```python
from build123d import *

# Parameters (mm, degrees)
EXTRUDE_1_DEPTH     = 58.3
CUT_EXTRUDE_1_DEPTH = 6.8
CUT_EXTRUDE_2_DEPTH = 54.3
SKETCH_5_R          = 2
CUT_EXTRUDE_4_DEPTH = 55
CHAMFER_2_SIZE      = 1
SKETCH_7_R          = 3.25
CUT_EXTRUDE_5_DEPTH = 1
SKETCH_8_R          = 1.25
CUT_EXTRUDE_6_DEPTH = 10
SKETCH_9_R          = 1
CUT_EXTRUDE_7_DEPTH = 10
SKETCH_11_W         = 6
SKETCH_11_H         = 1.5
CUT_EXTRUDE_8_DEPTH = 10


with BuildPart() as part:
    # Эскиз1 → Бобышка-Вытянуть1 (new body)
    with BuildSketch(Plane.XY):
        with BuildLine():
            Line((-3.4, 9.15), (3.4, 9.15))
            ThreePointArc((3.4, 9.15), (6.935533906, 7.685533906), (8.4, 4.15))
            Line((8.4, 4.15), (8.4, -4.15))
            Line((8.4, -4.15), (-8.4, -4.15))
            Line((-8.4, -4.15), (-8.4, 4.15))
            ThreePointArc((-8.4, 4.15), (-6.935533906, 7.685533906), (-3.4, 9.15))
        make_face()
    extrude(amount=EXTRUDE_1_DEPTH)

    # Эскиз2 → Вырез-Вытянуть1 (cut)
    with BuildSketch(Plane(origin=(0, 9.15, 0), x_dir=(1, 0, 0), z_dir=(0, 1, 0))):
        with BuildLine():
            Line((8.4, -19.65), (8.4, -2))
            Line((8.4, -2), (-8.4, -2))
            Line((-8.4, -2), (-8.4, -19.65))
            Line((-8.4, -19.65), (-6, -19.65))
            ThreePointArc((-6, -19.65), (-4.585786438, -20.235786438), (-4, -21.65))
            Line((-4, -21.65), (-4, -36.65))
            ThreePointArc((-4, -36.65), (-4.585786438, -38.064213562), (-6, -38.65))
            Line((-6, -38.65), (-8.4, -38.65))
            Line((-8.4, -38.65), (-8.4, -56.3))
            Line((-8.4, -56.3), (8.4, -56.3))
            Line((8.4, -56.3), (8.4, -38.65))
            Line((8.4, -38.65), (6, -38.65))
            ThreePointArc((6, -38.65), (4.585786438, -38.064213562), (4, -36.65))
            Line((4, -36.65), (4, -21.65))
            ThreePointArc((4, -21.65), (4.585786438, -20.235786438), (6, -19.65))
            Line((6, -19.65), (8.4, -19.65))
        make_face()
    extrude(amount=-CUT_EXTRUDE_1_DEPTH, mode=Mode.SUBTRACT)

    # Эскиз3 → Вырез-Вытянуть2 (cut)
    with BuildSketch(Plane(origin=(0, 0, 56.3), x_dir=(-1, 0, 0), z_dir=(0, 0, -1))):
        with BuildLine():
            Line((-7.4, 4.15), (-7.4, -3.15))
            Line((-7.4, -3.15), (7.4, -3.15))
            Line((7.4, -3.15), (7.4, 4.15))
            ThreePointArc((7.4, 4.15), (6.228427125, 6.978427125), (3.4, 8.15))
            Line((3.4, 8.15), (-3.4, 8.15))
            ThreePointArc((-3.4, 8.15), (-6.228427125, 6.978427125), (-7.4, 4.15))
        make_face()
    extrude(amount=CUT_EXTRUDE_2_DEPTH, mode=Mode.SUBTRACT)

    # Эскиз5 → Вырез-Вытянуть4 (cut)
    with BuildSketch(Plane(origin=(0, -3.15, 0), x_dir=(1, 0, 0), z_dir=(0, 1, 0))):
        with Locations(Location((0, -29.15, 0), (0, 0, 270))):
            Circle(SKETCH_5_R)
    extrude(amount=-CUT_EXTRUDE_4_DEPTH, mode=Mode.SUBTRACT)

    # Фаска2
    chamfer_2_edges = [part.edges().sort_by_distance(p)[0] for p in [
        (0, -3.15, 27.15),
    ]]
    chamfer(chamfer_2_edges, length=CHAMFER_2_SIZE - 0.0001)  # a hair under: the kernel refuses the full size

    # Эскиз7 → Вырез-Вытянуть5 (cut)
    with BuildSketch(Plane(origin=(0, 0, 0), x_dir=(-1, 0, 0), z_dir=(0, 0, -1))):
        with Locations((0, 3.85)):
            Circle(SKETCH_7_R)
    cut_extrude_5 = extrude(amount=-CUT_EXTRUDE_5_DEPTH, mode=Mode.SUBTRACT)

    # Эскиз8 → Вырез-Вытянуть6 (cut)
    with BuildSketch(Plane(origin=(0, 0, 0), x_dir=(-1, 0, 0), z_dir=(0, 0, -1))):
        with Locations((0, 3.85)):
            Circle(SKETCH_8_R)
    cut_extrude_6 = extrude(amount=-CUT_EXTRUDE_6_DEPTH, mode=Mode.SUBTRACT)

    # Эскиз9 → Вырез-Вытянуть7 (cut)
    with BuildSketch(Plane(origin=(0, 0, 0), x_dir=(-1, 0, 0), z_dir=(0, 0, -1))):
        with Locations((-5.4, -1.65)):
            Circle(SKETCH_9_R)
    cut_extrude_7 = extrude(amount=-CUT_EXTRUDE_7_DEPTH, mode=Mode.SUBTRACT)

    # Эскиз11 → Вырез-Вытянуть8 (cut)
    with BuildSketch(Plane(origin=(0, -3.15, 0), x_dir=(1, 0, 0), z_dir=(0, 1, 0))):
        with Locations((0, -2.75)):
            Rectangle(SKETCH_11_W, SKETCH_11_H)
    cut_extrude_8 = extrude(amount=-CUT_EXTRUDE_8_DEPTH, mode=Mode.SUBTRACT)

    # Зеркальное отражение1: Вырез-Вытянуть5, Вырез-Вытянуть6, Вырез-Вытянуть7, Вырез-Вытянуть8 across plane
    add(cut_extrude_5.mirror(Plane(origin=(0, 0, 29.15), x_dir=(1, 0, 0), z_dir=(0, 0, -1))), mode=Mode.SUBTRACT)
    add(cut_extrude_6.mirror(Plane(origin=(0, 0, 29.15), x_dir=(1, 0, 0), z_dir=(0, 0, -1))), mode=Mode.SUBTRACT)
    add(cut_extrude_7.mirror(Plane(origin=(0, 0, 29.15), x_dir=(1, 0, 0), z_dir=(0, 0, -1))), mode=Mode.SUBTRACT)
    add(cut_extrude_8.mirror(Plane(origin=(0, 0, 29.15), x_dir=(1, 0, 0), z_dir=(0, 0, -1))), mode=Mode.SUBTRACT)


solid = part.part
```
Work out the finished part from the listing and answer in its coordinate system (mm). A direction names the side the tool comes from. Round coordinates to 2 decimals unless told otherwise and drop trailing zeros. Loops run counter-clockwise (first coordinate to the right, second up) from the corner with the lowest first, then second, coordinate; pieces in that order, holes last. Notation, with made-up numbers: (75, -3.75) -> (100, -3.75) arc R25 cw to (100, 31.25) -> close; hole circle Ø7 at (15.5, -10.5). An arc over 180 degrees is marked (long way). Write each question's results on one line, items separated by ' | '. Start each with the question number.
1. Find the intervals of material crossed by probe 1 along Z at (x, y) = (-7.5, 6.5); probe 2 along X at (y, z) = (3.85, 56.7); probe 3 along Y at (x, z) = (0, 0.7), in increasing order. Write a range as from..to.
2. For a pull along X with two mould halves and no side action, classify faces 6 (the face through (-8, 2.35, 11)), 7 (the face through (6.9, 7.72, 57.29)), 8 (the face through (4.6, 8.38, 38.08)) as +X half, -X half, draft (parallel to the pull), parting line (faces both ways), or undercut.
3. Section C-C (y = -1.65) is taken. Determine the outline of the cut face in (x, z), plus the area to 3 significant figures.
4. Section B-B (x = 0) is taken. State how many separate pieces and enclosed holes the cut face has, plus the area to 3 significant figures.
5. Given pin 1 Ø3 at (x, y) = (-6, -1.5) entering from -Z; pin 2 Ø5 at (x, z) = (-6, 43) entering from +Y; pin 3 Ø1.5 at (x, z) = (-0.5, 20.5) entering from +Y; pin 4 Ø0.5 at (y, z) = (9, 27.5) entering from +X, each flat-ended and moving along its own axis, determine where each tip first touches the part or whether it passes through.
6. A tool of negligible diameter and unlimited length cuts with its end or side. For faces 1 (the face through (0.705, 0.677, 0.493)), 2 (the face through (-4.6, 8.38, 20.22)), 3 (the face through (0, 2, 57.3)), 4 (the face through (8, 2.35, 47)), 5 (the face through (3, -4, 56)), from which of +Z, -Z, +X, -X, +Y, -Y can it reach the whole face along a straight path? Write none if from no direction.
7. Section D-D (x = 5.4) is taken. Determine the outline of the cut face in (y, z).
Evaluation:
1) probe 1: z = 0..2, 19.65..38.65, 56.3..58.3 | probe 2: x = -8.4..-1.25, 1.25..8.4 | probe 3: y = -4.15..0.6, 7.1..9.15
2) face 6: draft | face 7: +X half | face 8: undercut
3) outline: (-8.4, 0) -> (4.4, 0) -> (4.4, 2) -> (-7.4, 2) -> (-7.4, 56.3) -> (4.4, 56.3) -> (4.4, 58.3) -> (-8.4, 58.3) -> close; (6.4, 0) -> (8.4, 0) -> (8.4, 58.3) -> (6.4, 58.3) -> (6.4, 56.3) -> (7.4, 56.3) -> (7.4, 2) -> (6.4, 2) -> close | area: 168 mm2
4) separate pieces: 6 | enclosed holes: 0 | area: 81.5 mm2
5) pin 1: stops at z = 0 | pin 2: stops at y = 2.35 | pin 3: stops at y = -3.15 | pin 4: stops at x = 5.36
6) face 1: -Z | face 2: +Y | face 3: +Z | face 4: +X, -X, +Y | face 5: +Y, -Y
7) outline: (-4.15, 0) -> (-2.65, 0) -> (-2.65, 2) -> (-3.15, 2) -> (-3.15, 56.3) -> (-2.65, 56.3) -> (-2.65, 58.3) -> (-4.15, 58.3) -> close; (-0.65, 0) -> (8.73, 0) -> (8.73, 2) -> (-0.65, 2) -> close; (-0.65, 56.3) -> (8.73, 56.3) -> (8.73, 58.3) -> (-0.65, 58.3) -> close; (7.61, 19.74) -> (8.73, 19.74) -> (8.73, 38.56) -> (7.61, 38.56) -> close
